Here's how the part is built. I have some questions about the finished solid (model axes, mm). Coordinates: 2 decimals unless noted, no trailing zeros. Write each loop counter-clockwise with the first axis right and the second up, starting at its lowest first coordinate (ties: lowest second). Pieces come first, ordered by that corner, then holes.
(1) Imagine slicing it at B-B, the plane z = 0. List the corners of the cut face in (x, y) for me, plus the area to 3 significant figures.
(2) Please list where these lines run through material, in increasing order: probe 1 along Y at (x, z) = (-105, -6.7); probe 2 along X at (y, z) = (5, -8.3); probe 3 along Z at (x, y) = (-75, 17.5).
(3) Imagine slicing it at C-C, the plane y = -25. List the corners of the cut face in (x, z) for me, plus the area to 3 significant figures.
(4) For pin 1 Ø3 at (x, y) = (-105, -5) entering from -Z; pin 2 Ø5 at (x, z) = (-75, 0) entering from +Y, each with a flat end and sliding along its axis, tell me the tip position at first contact or that it passes through.
(5) Imagine slicing it at A-A, the plane x = 75. List the corners of the cut face in (y, z) for me, plus the area to 3 significant figures.
(6) Thinking about a two-plate mould opening in X: for faces 1 (the flat face through (175, -1, 0)), 2 (the cylindrical face through (77.4, 0.9, -1.8)), 3 (the flat face through (-2, 1, 10)), which applies, released by +X, released by -X, zero draft, split by the parting line, or undercut?
```python
from build123d import *

# Parameters (mm, degrees)
F0_W     = 350
F0_H     = 130
F1_DEPTH = 10
F3_D     = 6
F5_D     = 3.5
F5_DEPTH = 5
F5_TIP   = 1.0515060833


with BuildPart() as f1:
    # F0 (on Top) → F1 (new body, symmetric)
    with BuildSketch(Plane.XY):
        Rectangle(F0_W, F0_H)
    extrude(amount=F1_DEPTH, both=True)

    # F3 (through all)
    with Locations(Plane.XZ.offset(65)):
        with Locations((-125, 0), (-75, 0), (75, 0), (125, 0)):
            Hole(F3_D / 2)

    # F5
    with Locations(Plane(origin=(0, 0, -10), x_dir=(1, 0, 0), z_dir=(0, 0, -1))):
        with Locations((-105, 5), (-105, -5), (-95, 0), (-5, 5), (-5, -5), (5, 0)):
            Hole(F5_D / 2, depth=F5_DEPTH)
            with Locations((0, 0, -(F5_DEPTH + F5_TIP / 2))):  # 118° drill point
                Cone(0, F5_D / 2, F5_TIP, mode=Mode.SUBTRACT)


solid = f1.part
```
Recorded:
1. outline: (-175, -65) - (-128, -65) - (-128, 65) - (-175, 65) - close; (-122, -65) - (-78, -65) - (-78, 65) - (-122, 65) - close; (-72, -65) - (72, -65) - (72, 65) - (-72, 65) - close; (78, -65) - (122, -65) - (122, 65) - (78, 65) - close; (128, -65) - (175, -65) - (175, 65) - (128, 65) - close
1. area: 42,400 mm2
2. probe 1: y = -65 to -6.75, -3.25 to 3.25, 6.75 to 65
2. probe 2: x = -175 to -106.75, -103.25 to -6.75, -3.25 to 175
2. probe 3: z = -10 to -3, 3 to 10
3. outline: (-175, -10) - (175, -10) - (175, 10) - (-175, 10) - close; hole circle Ø6 at (-125, 0); hole circle Ø6 at (-75, 0); hole circle Ø6 at (75, 0); hole circle Ø6 at (125, 0)
3. area: 6,890 mm2
4. pin 1: stops at z = -4.85
4. pin 2: passes through
5. outline: (-65, -10) - (65, -10) - (65, -3) - (-65, -3) - close; (-65, 3) - (65, 3) - (65, 10) - (-65, 10) - close
5. area: 1,820 mm2
6. face 1: released by +X
6. face 2: undercut
6. face 3: zero draft
